Geometry: final body of the model. Coordinates: model frame, mm. A direction names the side the tool comes from. Round coordinates to 2 decimals unless told otherwise and drop trailing zeros. Order: outer loops, then holes, each group sorted by start corner. A loop starts at its lowest first (then second) coordinate and runs counter-clockwise, first axis right, second up. Notation, with made-up numbers: M 37,-27.75 L 49,-27.75 A21 ccw 49,-7.75 Z; hole C 62,78.5 d8. An arc over 180 degrees is marked long. Put each result on its own line as item: value. Start each with the question number.
1) First-contact query: P1, Ø1.5, axis at x = -14, z = -54.5, coming from the +Y side; P2, Ø10, axis at x = -9, z = -14.5, coming from the +Y side. Flat tips, straight axial feed; report the tip coordinate or a pass-through.
2) Material intervals for probe 1 along Z at (x, y) = (-71, -204.5); probe 2 along X at (y, z) = (-194, -122); probe 3 along X at (y, z) = (25, -21), sorted ascending. Write a range as [from, to].
3) Section C-C, the plane z = -190. Return loops of the section in (x, y), then the cut area to 3 significant figures.
4) Section A-A, the plane y = 13.5. Return loops of the section in (x, z).
5) Access query for faces 1 (the flat face through (-9, -7.447, -15)), 2 (the cylindrical face through (-47.735, 39.546, -12.675)), 3 (the flat face through (-110, 42.553, -170)). Directions: +Z, -Z, +X, -X, +Y, -Y. A direction counts if a zero-diameter tool reaches every point of the face in a straight line with its end or side. Return the directions, or none.
6) Draft query along X for faces 4 (the flat face through (-10, -105, 0)), 5 (the flat face through (96.117, -110, -182)), 6 (the flat face through (-113.883, -110, -182)), 7 (the flat face through (86.117, -95, -193)). Return one class per face: pulls with the +X half, pulls with the -X half, needs draft (parallel to the pull), parting line crosses it, or undercut.
7) Section B-B, the plane x = -86.5. Return loops of the section in (y, z), then the cut area to 3 significant figures.
8) Section D-D, the plane y = -179.5. Return loops of the section in (x, z).
from build123d import *

# Parameters (mm, degrees)
ESQUISSE1_W             = 210
ESQUISSE1_H             = 300
BOSS_EXTRU_1_DEPTH      = 370
ESQUISSE2_W             = 190
ESQUISSE2_H             = 330
ENL_V_MAT_EXTRU_1_DEPTH = 280
ESQUISSE5_W             = 72
ESQUISSE5_H             = 25
ENL_V_MAT_EXTRU_4_DEPTH = 35
ESQUISSE6_W             = 72
ESQUISSE6_H             = 20
ENL_V_MAT_EXTRU_5_DEPTH = 15
CONG_5_R                = 10
CONG_6_R                = 10
CONG_7_R                = 10


with BuildPart() as part:
    # Esquisse1 → Boss.-Extru.1 (new body)
    with BuildSketch(Plane.XY):
        with Locations((-8.883179232, -107.447368421)):
            Rectangle(ESQUISSE1_W, ESQUISSE1_H)
    extrude(amount=-BOSS_EXTRU_1_DEPTH)

    # Esquisse2 → Enlèv. mat.-Extru.1 (cut)
    with BuildSketch(Plane(origin=(0, 42.552631579, 0), x_dir=(1, 0, 0), z_dir=(0, 1, 0))):
        with Locations((-8.883179232, 195)):
            Rectangle(ESQUISSE2_W, ESQUISSE2_H)
    extrude(amount=-ENL_V_MAT_EXTRU_1_DEPTH, mode=Mode.SUBTRACT)

    # Esquisse5 → Enlèv. mat.-Extru.4 (cut)
    with BuildSketch(Plane(origin=(0, 42.552631579, 0), x_dir=(1, 0, 0), z_dir=(0, 1, 0))):
        with Locations((-8.883179232, 12.5)):
            Rectangle(ESQUISSE5_W, ESQUISSE5_H)
    extrude(amount=-ENL_V_MAT_EXTRU_4_DEPTH, mode=Mode.SUBTRACT)

    # Esquisse6 → Enlèv. mat.-Extru.5 (cut)
    with BuildSketch(Plane(origin=(0, 7.552631579, 0), x_dir=(1, 0, 0), z_dir=(0, 1, 0))):
        with Locations((-8.883179232, 15)):
            Rectangle(ESQUISSE6_W, ESQUISSE6_H)
    extrude(amount=-ENL_V_MAT_EXTRU_5_DEPTH, mode=Mode.SUBTRACT)

    # Congé5
    cong_5_edges = [part.edges().sort_by_distance(p)[0] for p in [
        (27.116820768, 42.552631579, -12.5),
    ]]
    fillet(cong_5_edges, radius=CONG_5_R)

    # Congé6
    cong_6_edges = [part.edges().sort_by_distance(p)[0] for p in [
        (-44.883179232, 42.552631579, -12.5),
    ]]
    fillet(cong_6_edges, radius=CONG_6_R)

    # Congé7
    # the kernel refuses this fillet: 10 mm, written as the material it takes off along each edge
    with BuildSketch(Plane(origin=(27.116820768, 7.552631579, -5), x_dir=(0, -1, 0), z_dir=(-1, 0, 0))) as cong_7_piece_1:
        with BuildLine():
            CenterArc((8.660254038, 10), CONG_7_R, 210, 60)
            Line((0, 5), (-0.173205081, 4.9))
            ThreePointArc((-0.173205081, 4.9), (-0.2, 2.5), (-0.2, 0))
            Line((-0.2, 0), (0, -0.2))
            Line((0, -0.2), (8.660254038, -0.2))
            Line((8.660254038, -0.2), (8.660254038, 0))
        make_face()
    extrude(amount=72, mode=Mode.SUBTRACT)


solid = part.part
Result sheet:
1. P1: stops at y = -237.45
1. P2: stops at y = -7.45
2. probe 1: z = [-370, -360], [-30, 0]
2. probe 2: x = [-113.88, -103.88], [86.12, 96.12]
2. probe 3: x = [-113.88, -44.88], [27.12, 96.12]
3. outline: M -113.88,-257.45 L 96.12,-257.45 L 96.12,42.55 L 86.12,42.55 L 86.12,-237.45 L -103.88,-237.45 L -103.88,42.55 L -113.88,42.55 Z
3. area: 9,800 mm2
4. outline: M -113.88,-370 L 96.12,-370 L 96.12,0 L 27.12,0 L 27.12,-25 L -44.88,-25 L -44.88,0 L -113.88,0 Z; hole M -103.88,-360 L 86.12,-360 L 86.12,-30 L -103.88,-30 Z
5. face 1: +Y
5. face 2: +Z, +Y
5. face 3: +Z, -Z, +X, -X, +Y
6. face 4: needs draft
6. face 5: pulls with the +X half
6. face 6: pulls with the -X half
6. face 7: undercut
7. outline: M -257.45,-370 L 42.55,-370 L 42.55,-360 L -237.45,-360 L -237.45,-30 L 42.55,-30 L 42.55,0 L -257.45,0 Z
7. area: 18,600 mm2
8. outline: M -113.88,-370 L 96.12,-370 L 96.12,0 L -113.88,0 Z; hole M -103.88,-360 L 86.12,-360 L 86.12,-30 L -103.88,-30 Z
